Part model, mm, in its own coordinate system. A direction names the side the tool comes from. Round coordinates to 2 decimals unless told otherwise and drop trailing zeros. Loops run counter-clockwise (first coordinate to the right, second up) from the corner with the lowest first, then second, coordinate; pieces in that order, holes last. Notation, with made-up numbers: (-12.5, 81.5) -> (29.5, 81.5) arc R35 ccw to (29.5, 117.5) -> close; hole circle Ø4 at (-33.75, 60.25). An arc over 180 degrees is marked (long way). Answer as CSV lines item,"result".
from build123d import *

# Parameters (mm, degrees)
F1_DEPTH = 25.4
F3_DEPTH = 25.4
F5_DEPTH = 25.4


with BuildPart() as f1:
    # F0 (on Front) → F1 (new body)
    with BuildSketch(Plane.XZ):
        Polygon((-2.625628, 15.450482), (-9.327945, 24.465393), (-19.639778, 28.921377), (-30.798078, 27.624455), (-39.81299, 20.922138), (-44.268973, 10.610306), (-42.972052, -0.547995), (-36.269735, -9.562907), (-25.957902, -14.01889), (-14.799602, -12.721969), (-5.78469, -6.019652), (-1.328707, 4.292181), align=None)
    extrude(amount=F1_DEPTH)

    # F2 (on face) → F3 (cut)
    with BuildSketch(Plane.XZ.offset(25.4)):
        Polygon((-42.977218, 21.73793), (-46.744515, 11.969563), (-36.401212, 13.591172), align=None)
    extrude(amount=-F3_DEPTH, mode=Mode.SUBTRACT)

    # F4 (on face) → F5 (cut)
    with BuildSketch(Plane.XZ.offset(25.4)):
        Polygon((-31.939655, 27.643172), (-39.482275, 20.382153), (-29.422739, 17.480562), align=None)
    extrude(amount=-F5_DEPTH, mode=Mode.SUBTRACT)


solid = f1.part
Q1. Saw through at C-C, the plane z = 16. Write the cut outline in (x, y).
Geometry results:
outline,"(-38.35, -25.4) -> (-3.03, -25.4) -> (-3.03, 0) -> (-38.35, 0) -> close"
Q2. Two-plate mould, pull along Z, no slides. Class faces 4 (the face through (-39.67, -12.52, -4.99)), 5 (the face through (-5.93, -12.522, 19.895)), 6 (the face through (-34.52, -12.88, 18.95)): pulls with the +Z half, pulls with the -Z half, needs draft (parallel to the pull), parting line crosses it, or undercut.
Geometry results:
face 4,"pulls with the -Z half"
face 5,"pulls with the +Z half"
face 6,"undercut"
Q3. Drill centre lines: line 1 along Z through (x, y) = (-38, -4.5); line 2 along X through (y, z) = (-8.5, 14); line 3 along Z through (x, y) = (-6, -5.5). Where is each one in solid material? Low to high.
Geometry results:
line 1,"-7.24 to 13.34, 15.57 to 19.95, 21.81 to 22.27"
line 2,"-36.73 to -2.46"
line 3,"-6.18 to 19.99"
Q4. Saw through at A-A, the plane y = -2.25. Write the cut outline in (x, z).
Geometry results:
outline,"(-44.27, 10.61) -> (-42.97, -0.55) -> (-36.27, -9.56) -> (-25.96, -14.02) -> (-14.8, -12.72) -> (-5.78, -6.02) -> (-1.33, 4.29) -> (-2.63, 15.45) -> (-9.33, 24.47) -> (-19.64, 28.92) -> (-30.8, 27.62) -> (-31.76, 26.91) -> (-29.42, 17.48) -> (-39.48, 20.38) -> (-35.9, 23.83) -> (-39.81, 20.92) -> (-40.69, 18.9) -> (-36.4, 13.59) -> (-43.46, 12.48) -> close"
Q5. Drop flat-ended pins along their axis: P1, Ø8, axis at x = -33.5, y = -10.5, coming from the -Z side; P2, Ø10, axis at y = -20.5, z = -0.5, coming from the +X side; P3, Ø5, axis at x = -16.5, y = -19, coming from the +Z side; P4, Ø1, axis at y = -8.5, z = 11.5, coming from the -X side. Give the stop position or say it passes through.
Geometry results:
P1,"z = -12.49"
P2,"x = -1.33"
P3,"z = 28.64"
P4,"x = -44.1"
Q6. Which spindle directions (+Z, -Z, +X, -X, +Y, -Y) get a long thin tool onto all of the face, cutting with end or side? Do faces 1 (the face through (-14.41, -12.52, 26.66)), 2 (the face through (-30.574, -12.878, 22.13)), 3 (the face through (-38.514, -12.878, 16.209)). Say none if no direction does.
Geometry results:
face 1,"+Z, +X, +Y, -Y"
face 2,"+Y, -Y"
face 3,"-X, +Y, -Y"
Q7. Saw through at B-B, the plane x = -10.5. Write the cut outline in (y, z), then the cut area to 3 significant figures.
Geometry results:
outline,"(-25.4, -9.53) -> (0, -9.53) -> (0, 24.97) -> (-25.4, 24.97) -> close"
area,"876 mm2"
